Read the model definition and answer for the solid it produces. Units are mm, in the model's axes. Face numbers are marked on the shaded views. Coordinates: 2 decimals unless noted, no trailing zeros. Write each loop counter-clockwise with the first axis right and the second up, starting at its lowest first coordinate (ties: lowest second). Pieces come first, ordered by that corner, then holes. Notation, with made-up numbers: (1.25, 44.25) -> (52.25, 44.25) arc R33 cw to (52.25, 80.25) -> close; hole circle Ø5 at (15.5, -11). An arc over 180 degrees is marked (long way). One line per item, written item: value. Start each with the question number.
from build123d import *

# Parameters (mm, degrees)
SKETCH_W  = 100
SKETCH_H  = 200
SKETCH_R  = 36.5
PAD_DEPTH = 12


with BuildPart() as part:
    # Sketch → Pad (new body)
    with BuildSketch(Plane.XY):
        with Locations((50, 100)):
            Rectangle(SKETCH_W, SKETCH_H)
        with Locations((50, 150)):
            Circle(SKETCH_R, mode=Mode.SUBTRACT)
        with BuildLine():
            Line((18, 20), (82, 20))
            ThreePointArc((82, 20), (84.12132, 20.87868), (85, 23))
            Line((85, 23), (85, 27))
            ThreePointArc((85, 27), (84.12132, 29.12132), (82, 30))
            Line((82, 30), (18, 30))
            ThreePointArc((18, 30), (15.87868, 29.12132), (15, 27))
            Line((15, 27), (15, 23))
            ThreePointArc((15, 23), (15.87868, 20.87868), (18, 20))
        make_face(mode=Mode.SUBTRACT)
    extrude(amount=PAD_DEPTH)


solid = part.part
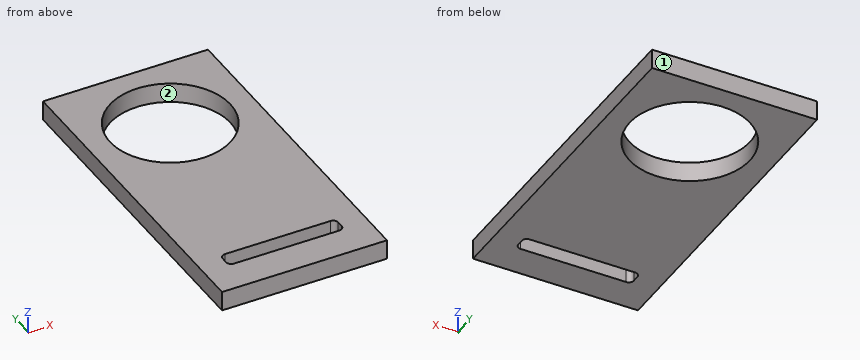
1. For a pull along X with two mould halves and no side action, classify the marked faces 1 and 2 as +X half, -X half, draft (parallel to the pull), parting line (faces both ways), or undercut.
2. A cutting plane is placed at B-B on x = 50. Give the vertices of the cut face in (y, z), then the cut area to 3 significant figures.
3. Given pin 1 (4.5 mm diameter, centred on y = 25, z = 9, fed in from -X), flat-ended and moving along its own axis, determine where the tip first touches the part or whether it passes through.
4. A cutting plane is placed at D-D on x = 29. Give the vertices of the cut face in (y, z).
5. A cutting plane is placed at A-A on z = 5.5. Give the vertices of the cut face in (x, y).
6. A cutting plane is placed at C-C on y = 150. Give the vertices of the cut face in (x, z), then the cut area to 3 significant figures.
7. Find the intervals of material crossed by probe 1 along Y at (x, z) = (50, 9); probe 2 along Y at (x, z) = (75, 6); probe 3 along X at (y, z) = (134.5, 4.5), in increasing order. Write a range as from..to.
Derived:
1. face 1: draft
1. face 2: undercut
2. outline: (0, 0) -> (20, 0) -> (20, 12) -> (0, 12) -> close; (30, 0) -> (113.5, 0) -> (113.5, 12) -> (30, 12) -> close; (186.5, 0) -> (200, 0) -> (200, 12) -> (186.5, 12) -> close
2. area: 1,400 mm2
3. pin 1: stops at x = 0
4. outline: (0, 0) -> (20, 0) -> (20, 12) -> (0, 12) -> close; (30, 0) -> (120.15, 0) -> (120.15, 12) -> (30, 12) -> close; (179.85, 0) -> (200, 0) -> (200, 12) -> (179.85, 12) -> close
5. outline: (0, 0) -> (100, 0) -> (100, 200) -> (0, 200) -> close; hole circle Ø73 at (50, 150); hole (15, 23) arc R3 ccw to (18, 20) -> (82, 20) arc R3 ccw to (85, 23) -> (85, 27) arc R3 ccw to (82, 30) -> (18, 30) arc R3 ccw to (15, 27) -> close
6. outline: (0, 0) -> (13.5, 0) -> (13.5, 12) -> (0, 12) -> close; (86.5, 0) -> (100, 0) -> (100, 12) -> (86.5, 12) -> close
6. area: 324 mm2
7. probe 1: y = 0..20, 30..113.5, 186.5..200
7. probe 2: y = 0..20, 30..123.41, 176.59..200
7. probe 3: x = 0..16.95, 83.05..100
